Source: CAD feature listing. Evaluate the final solid. Frame: model axes, mm. Face numbers are marked on the shaded views. A direction names the side the tool comes from. Round coordinates to 2 decimals unless told otherwise and drop trailing zeros. Loops run counter-clockwise (first coordinate to the right, second up) from the corner with the lowest first, then second, coordinate; pieces in that order, holes last. Notation, with made-up numbers: M 43.25,54.5 L 66.25,54.5 A16 cw 66.25,73.5 Z; hole C 46.5,72.25 d1. An arc over 180 degrees is marked long. Answer as a JSON object with one key per item and string values.
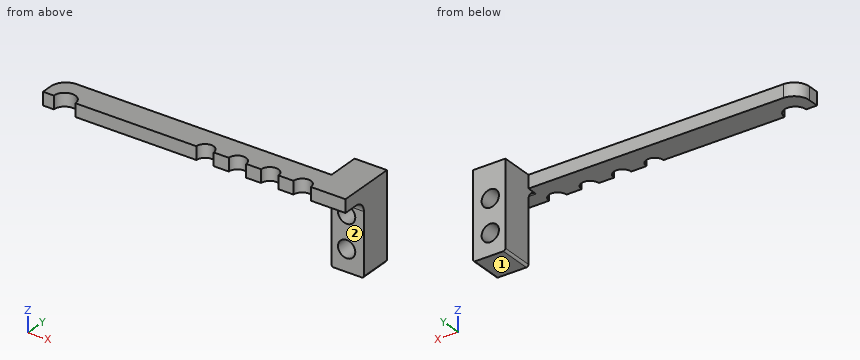
from build123d import *

# Parameters (mm, degrees)
F1_DEPTH = 6
F2_R     = 7
F3_W     = 15
F3_H     = 34
F3_H_2   = 6
F4_DEPTH = 15
F5_R     = 4
F6_DEPTH = 25
F7_R     = 4.99999
F8_R     = 1


# Not quite as in the source:
# - a fillet or chamfer is up to 0.001 mm smaller than in the source, because OpenCascade refuses the exact size


with BuildPart() as f1:
    # F0 (on Top) → F1 (new body)
    with BuildSketch(Plane.XY):
        with BuildLine():
            ThreePointArc((-70, 0), (-65, 5), (-60, 0))
            Line((-60, 0), (-4, 0))
            ThreePointArc((-4, 0), (0, 4), (4, 0))
            Line((4, 0), (11, 0))
            ThreePointArc((11, 0), (15, 4), (19, 0))
            Line((19, 0), (26, 0))
            ThreePointArc((26, 0), (30, 4), (34, 0))
            Line((34, 0), (41, 0))
            ThreePointArc((41, 0), (45, 4), (49, 0))
            Line((49, 0), (65, 0))
            Line((65, 0), (65, 12))
            Line((65, 12), (-75, 12))
            Line((-75, 12), (-75, 0))
            Line((-75, 0), (-70, 0))
        make_face()
    extrude(amount=F1_DEPTH)

    # F2
    f2_edges = [f1.edges().sort_by_distance(p)[0] for p in [
        (-75, 12, 3),
    ]]
    fillet(f2_edges, radius=F2_R)

    # F3 (on face) → F4 (join)
    with BuildSketch(Plane(origin=(0, 12, 0), x_dir=(-1, 0, 0), z_dir=(0, 1, 0))):
        with Locations((-57.5, -17)):
            Rectangle(F3_W, F3_H)
        with Locations((-57.5, 3)):
            Rectangle(F3_W, F3_H_2)
    extrude(amount=F4_DEPTH)

    # F5 (on face) → F6 (cut)
    with BuildSketch(Plane.XZ.offset(-12)):
        with Locations((57, -9)):
            Circle(F5_R)
        with Locations((57, -24)):
            Circle(F5_R)
    extrude(amount=-F6_DEPTH, mode=Mode.SUBTRACT)

    # F7 (radius 5 in the source; OpenCascade refuses exactly that, so slightly less here)
    f7_edges = [f1.edges().sort_by_distance(p)[0] for p in [
        (57.5, 12, 0),
    ]]
    fillet(f7_edges, radius=F7_R)

    # F8
    f8_edges = [f1.edges().sort_by_distance(p)[0] for p in [
        (65, 19.5, -34),
        (50, 19.5, -34),
    ]]
    fillet(f8_edges, radius=F8_R)


solid = f1.part
Item 1: Contact query for flat-ended pins moving along their axis: pin 1 Ø2 at (y, z) = (14.5, -15) entering from -X; pin 2 Ø6 at (x, y) = (-14, 7.5) entering from -Z; pin 3 Ø5 at (x, z) = (-41, 0.5) entering from +Y. Output: stop coordinate, or through.
Answer sheet:
{"pin 1": "stops at x = 50", "pin 2": "stops at z = 0", "pin 3": "stops at y = 12"}
Item 2: Section A-A on z = -24. Return the cut outline in (x, y), then the cut area to 3 significant figures.
Answer sheet:
{"outline": "M 50,12 L 53,12 L 53,27 L 50,27 Z; M 61,12 L 65,12 L 65,27 L 61,27 Z", "area": "105 mm²"}
Item 3: Section C-C on y = 25.25. Return the cut outline in (x, z), then the cut area to 3 significant figures.
Answer sheet:
{"outline": "M 50,-33 A1 ccw 51,-34 L 64,-34 A1 ccw 65,-33 L 65,6 L 50,6 Z; hole C 57,-24 d8; hole C 57,-9 d8", "area": "499 mm²"}
Item 4: Access query for the marked faces 1 and 2. Directions: +Z, -Z, +X, -X, +Y, -Y. A direction counts if a zero-diameter tool reaches every point of the face in a straight line with its end or side. Return the directions, or none.
Answer sheet:
{"face 1": "-Z, +X, -X, +Y, -Y", "face 2": "-Z, +X, -X, -Y"}
Item 5: Line query: probe 1 along Z at (x, y) = (57, 21.25); probe 2 along X at (y, z) = (21.5, -18); probe 3 along X at (y, z) = (25.75, -25). Output: solid intervals per line, ascending. Write a range as from..to.
Answer sheet:
{"probe 1": "z = -34..-28, -20..-13, -5..6", "probe 2": "x = 50..65", "probe 3": "x = 50..53.13, 60.87..65"}
Item 6: Section D-D on z = 2. Return the cut outline in (x, y), then the cut area to 3 significant figures.
Answer sheet:
{"outline": "M -75,0 L -70,0 A5 cw -60,0 L -4,0 A4 cw 4,0 L 11,0 A4 cw 19,0 L 26,0 A4 cw 34,0 L 41,0 A4 cw 49,0 L 65,0 L 65,27 L 50,27 L 50,12 L -68,12 A7 ccw -75,5 Z", "area": "1,750 mm²"}
Item 7: Section B-B on x = 57. Give the number of separate pieces and of enclosed holes in the cut face, then the cut area to 3 significant figures.
Answer sheet:
{"separate pieces": "3", "enclosed holes": "0", "area": "437 mm²"}
